```python
from build123d import *

# Parameters (mm, degrees)
EXTRUDE_1_DEPTH     = 40
SKETCH_2_R          = 10
SKETCH_2_R_2        = 1.5
CUT_EXTRUDE_1_DEPTH = 40
SKETCH_3_R          = 1.5
CUT_EXTRUDE_2_DEPTH = 68.594378464


with BuildPart() as part:
    # Эскиз1 → Бобышка-Вытянуть1 (new body)
    with BuildSketch(Plane(origin=(0, 0, 0), x_dir=(1, 0, 0), z_dir=(0, 1, 0))):
        Polygon((0, 0), (40, 0), (40, 3), (3, 3), (3, 40), (0, 40), align=None)
    extrude(amount=EXTRUDE_1_DEPTH)

    # Эскиз2 → Вырез-Вытянуть1 (cut)
    with BuildSketch(Plane(origin=(3, 0, 0), x_dir=(0, 0, -1), z_dir=(1, 0, 0))):
        with Locations((21.5, 20)):
            Circle(SKETCH_2_R)
        with Locations((30.5, 29)):
            Circle(SKETCH_2_R_2)
        with Locations((30.5, 11)):
            Circle(SKETCH_2_R_2)
        with Locations((12.5, 11)):
            Circle(SKETCH_2_R_2)
        with Locations((12.5, 29)):
            Circle(SKETCH_2_R_2)
    extrude(amount=-CUT_EXTRUDE_1_DEPTH, mode=Mode.SUBTRACT)

    # Эскиз3 → Вырез-Вытянуть2 (cut, through all)
    with BuildSketch(Plane(origin=(0, 0, -3), x_dir=(-1, 0, 0), z_dir=(0, 0, -1))):
        with Locations((-30, 30)):
            Circle(SKETCH_3_R)
        with Locations((-12.679491924, 20)):
            Circle(SKETCH_3_R)
        with Locations((-30, 10)):
            Circle(SKETCH_3_R)
    extrude(amount=-CUT_EXTRUDE_2_DEPTH, mode=Mode.SUBTRACT)


solid = part.part
```
Could you check a few things on this model? Use its own coordinates, in mm. A direction names the side the tool comes from. Round coordinates to 2 decimals unless told otherwise and drop trailing zeros. Loops run counter-clockwise (first coordinate to the right, second up) from the corner with the lowest first, then second, coordinate; pieces in that order, holes last. Notation, with made-up numbers: (-11, -20) - (-5, -20) arc R30 cw to (-5, 15) - close; hole circle Ø1 at (-0.75, 37). An arc over 180 degrees is marked (long way). Answer in a Markdown table with one row per item. Add a question column.
(1) If we section it at B-B (z = -21.5): Please give me the cut outline in (x, y), plus the area to 3 significant figures.
(2) If we mould it in two halves opening along Z, with no side actions, what happens to faces 3 (the face through (31.5, 10.07, -1.52)), 4 (the face through (1.52, 23, -31.04)), 5 (the face through (20, 20, 0)), 6 (the face through (2, 11, -29))? For each: pulls with the +Z half, pulls with the -Z half, needs draft (parallel to the pull), parting line crosses it, or undercut.
(3) I'm going to push flat-ended pins straight in: pin 1 (10 mm diameter, centred on x = 26.5, y = 19, fed in from -Z); pin 2 (3 mm diameter, centred on y = 7, z = -16.5, fed in from +X); pin 3 (2.5 mm diameter, centred on x = 30, y = 10, fed in from +Z). Where does each tip first touch, or does it pass through?
(4) For faces 1 (the face through (22, 20, -3)), 2 (the face through (1.521, 30.487, -12.305)), which set-ups out of +Z, -Z, +X, -X, +Y, -Y let a thin tool reach every point of the face, with its end or its side?
(5) If we section it at D-D (z = -15.5): Please give me the cut outline in (x, y), plus the area to 3 significant figures.
(6) I need wall thicknesses on line 1 along Y through (x, z) = (0.7, -30.5); line 2 along Z through (x, y) = (13, 4); line 3 along X through (y, z) = (9.5, -7). Which ranges of each line are inside material? Lowest first, please.
(7) If we section it at A-A (x = 30): Please give me the cut outline in (y, z).
(8) If we section it at C-C (y = 24): Please give me the cut outline in (x, z).
Model answer:
| question | item | result |
|---|---|---|
| 1 | outline | (0, 0) - (3, 0) - (3, 10) - (0, 10) - close; (0, 30) - (3, 30) - (3, 40) - (0, 40) - close |
| 1 | area | 60.0 mm² |
| 2 | face 3 | needs draft |
| 2 | face 4 | undercut |
| 2 | face 5 | pulls with the +Z half |
| 2 | face 6 | undercut |
| 3 | pin 1 | stops at z = -3 |
| 3 | pin 2 | stops at x = 3 |
| 3 | pin 3 | passes through |
| 4 | face 1 | -Z, +X, +Y, -Y |
| 4 | face 2 | +X, -X |
| 5 | outline | (0, 0) - (3, 0) - (3, 12) - (0, 12) - close; (0, 28) - (3, 28) - (3, 40) - (0, 40) - close |
| 5 | area | 72.0 mm² |
| 6 | line 1 | y = 0 to 9.5, 12.5 to 15.64, 24.36 to 27.5, 30.5 to 40 |
| 6 | line 2 | z = -3 to 0 |
| 6 | line 3 | x = 0 to 3 |
| 7 | outline | (0, -3) - (8.5, -3) - (8.5, 0) - (0, 0) - close; (11.5, -3) - (28.5, -3) - (28.5, 0) - (11.5, 0) - close; (31.5, -3) - (40, -3) - (40, 0) - (31.5, 0) - close |
| 8 | outline | (0, -40) - (3, -40) - (3, -30.67) - (0, -30.67) - close; (0, -12.33) - (3, -12.33) - (3, -3) - (40, -3) - (40, 0) - (0, 0) - close |
